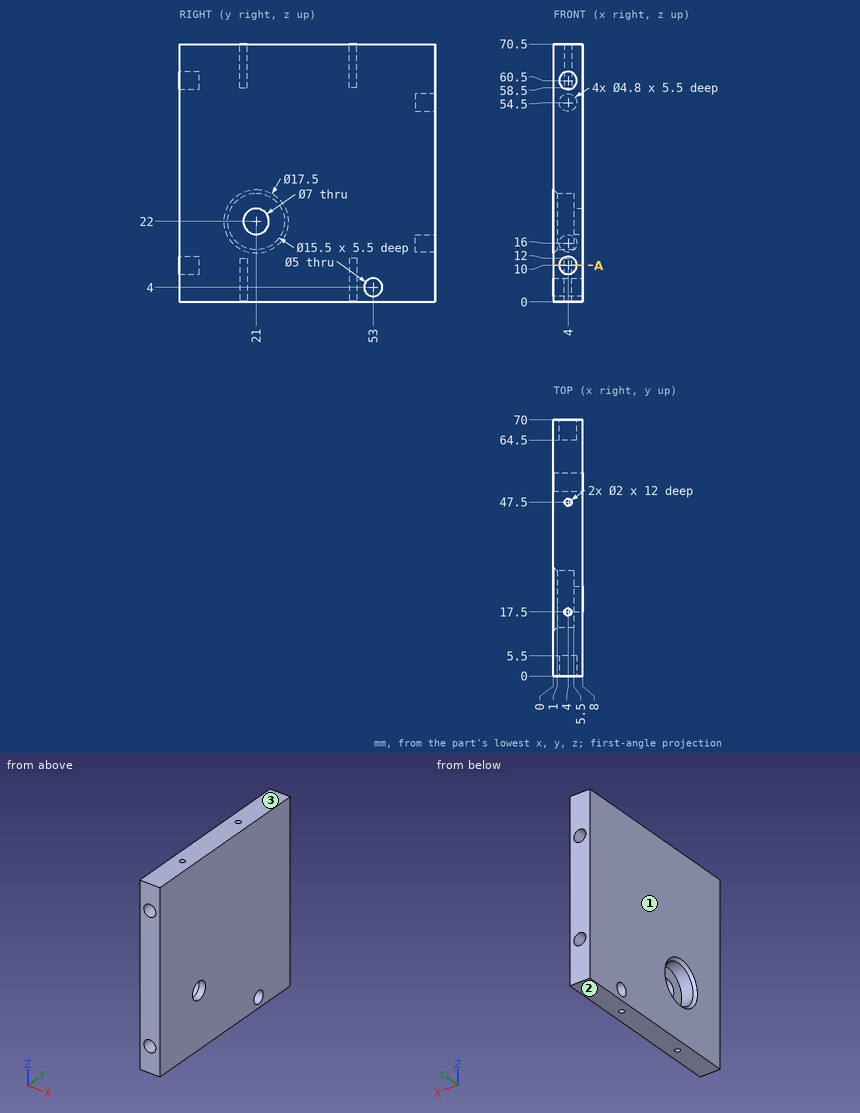
Design review of the part shown in the three views and the two pictorial views. Dimensions are in mm from the part's minimum x, y and z. Coordinates: 2 decimals unless noted, no trailing zeros. Order: outer loops, then holes, each group sorted by start corner. A loop starts at its lowest first (then second) coordinate and runs counter-clockwise, first axis right, second up.
Item 1: The part is to be moulded in two halves that separate along Z. For the marked faces 1, 2 and 3, say which applies: pulls with the +Z half, pulls with the -Z half, needs draft (parallel to the pull), parting line crosses it, or undercut.
Item 2: Take a section at A-A, the plane z = 10. Write out the cut boundary in (x, y).
Item 3: For line 1 (Y direction, x = 4, z = 8.75); line 2 (Y direction, x = 4, z = 68); line 3 (Z direction, x = 7.45, y = 21), list the stretches that pass through material, from the lowest coordinate up.
Item 4: For pin 1 Ø1.8 at (x, y) = (4, 17.5) entering from -Z; pin 2 Ø4 at (y, z) = (21, 22) entering from +X; pin 3 Ø1.4 at (x, z) = (4, 17) entering from +Y, all flat-tipped, find the tip position at first contact; note any pin that passes through.
The answers:
1. face 1: needs draft
1. face 2: pulls with the -Z half
1. face 3: pulls with the +Z half
2. outline: (0, 0) - (1.6, 0) - (1.6, 5.5) - (6.4, 5.5) - (6.4, 0) - (8, 0) - (8, 70) - (0, 70) - close; hole circle Ø2 at (4, 17.5); hole circle Ø2 at (4, 47.5)
3. line 1: y = 5.5 to 16.5, 18.5 to 46.5, 48.5 to 70
3. line 2: y = 0 to 16.5, 18.5 to 46.5, 48.5 to 70
3. line 3: z = 0 to 18.5, 25.5 to 70.5
4. pin 1: stops at z = 12
4. pin 2: passes through
4. pin 3: stops at y = 64.5
